The model under review builds one solid part; all positions refer to its coordinate system, in mm. Coordinates: 2 decimals unless noted, no trailing zeros. Write each loop counter-clockwise with the first axis right and the second up, starting at its lowest first coordinate (ties: lowest second). Pieces come first, ordered by that corner, then holes. Notation, with made-up numbers: M 70,19.25 L 117,19.25 A28 ccw 117,39.25 Z; hole C 50,66 d8. An arc over 180 degrees is marked long. Answer as a JSON object with one key per item and string values.
```python
from build123d import *

# Parameters (mm, degrees)
SKETCH1_W           = 150
SKETCH1_H           = 100
SKETCH1_R           = 2.5
SKETCH1_R_2         = 11.5
SKETCH1_R_3         = 1.5
SKETCH1_W_2         = 60
SKETCH1_H_2         = 45
BOSS_EXTRUDE1_DEPTH = 8
FILLET2_R           = 5
FILLET4_R           = 3


with BuildPart() as part:
    # Sketch1 → Boss-Extrude1 (new body)
    with BuildSketch(Plane(origin=(0, 0, 0), x_dir=(1, 0, 0), z_dir=(0, 1, 0))):
        Rectangle(SKETCH1_W, SKETCH1_H)
        with Locations(Location((-65, 40, 0), (0, 0, 270))):
            Circle(SKETCH1_R, mode=Mode.SUBTRACT)
        with Locations(Location((0, 40, 0), (0, 0, 270))):
            Circle(SKETCH1_R, mode=Mode.SUBTRACT)
        with Locations(Location((65, 40, 0), (0, 0, 270))):
            Circle(SKETCH1_R, mode=Mode.SUBTRACT)
        with Locations(Location((0, -40, 0), (0, 0, 270))):
            Circle(SKETCH1_R, mode=Mode.SUBTRACT)
        with Locations(Location((65, -40, 0), (0, 0, 270))):
            Circle(SKETCH1_R, mode=Mode.SUBTRACT)
        with Locations(Location((-65, -40, 0), (0, 0, 270))):
            Circle(SKETCH1_R, mode=Mode.SUBTRACT)
        with Locations(Location((-32.5, 0, 0), (0, 0, 270))):
            Circle(SKETCH1_R_2, mode=Mode.SUBTRACT)
        with Locations(Location((-50, 17.5, 0), (0, 0, 270))):
            Circle(SKETCH1_R_3, mode=Mode.SUBTRACT)
        with Locations(Location((-15, 17.5, 0), (0, 0, 270))):
            Circle(SKETCH1_R_3, mode=Mode.SUBTRACT)
        with Locations(Location((-15, -17.5, 0), (0, 0, 270))):
            Circle(SKETCH1_R_3, mode=Mode.SUBTRACT)
        with Locations(Location((-50, -17.5, 0), (0, 0, 270))):
            Circle(SKETCH1_R_3, mode=Mode.SUBTRACT)
        with Locations((27.5, 0)):
            Rectangle(SKETCH1_W_2, SKETCH1_H_2, mode=Mode.SUBTRACT)
    extrude(amount=BOSS_EXTRUDE1_DEPTH)

    # Fillet2
    fillet2_edges = [part.edges().sort_by_distance(p)[0] for p in [
        (-75, 4, 50),
        (-75, 4, -50),
        (75, 4, -50),
        (75, 4, 50),
    ]]
    fillet(fillet2_edges, radius=FILLET2_R)

    # Fillet4
    fillet4_edges = [part.edges().sort_by_distance(p)[0] for p in [
        (57.5, 4, 22.5),
        (57.5, 4, -22.5),
        (-2.5, 4, -22.5),
        (-2.5, 4, 22.5),
    ]]
    fillet(fillet4_edges, radius=FILLET4_R)


solid = part.part
```
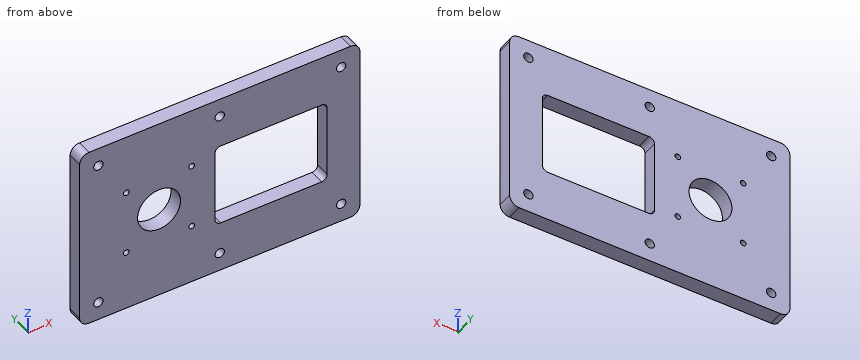
(1) Add section D-D on x = 65. Give the boundary of the cut face in (y, z), and give its area (3 significant figures).
Results list:
{"outline": "M 0,-50 L 8,-50 L 8,-42.5 L 0,-42.5 Z; M 0,-37.5 L 8,-37.5 L 8,37.5 L 0,37.5 Z; M 0,42.5 L 8,42.5 L 8,50 L 0,50 Z", "area": "720 mm²"}
(2) Wall thickness on line 1 along X through (y, z) = (2.5, 0); line 2 along X through (y, z) = (1.5, -40); line 3 along X through (y, z) = (7, 12.5): over which ranges is each line inside the solid? List them lowest first. Write a range as from..to.
Results list:
{"line 1": "-75..-44, -21..-2.5, 57.5..75", "line 2": "-75..-67.5, -62.5..-2.5, 2.5..62.5, 67.5..75", "line 3": "-75..-2.5, 57.5..75"}
(3) Add section A-A on z = 40. Give the boundary of the cut face in (x, y), and give its area (3 significant figures).
Results list:
{"outline": "M -75,0 L -67.5,0 L -67.5,8 L -75,8 Z; M -62.5,0 L -2.5,0 L -2.5,8 L -62.5,8 Z; M 2.5,0 L 62.5,0 L 62.5,8 L 2.5,8 Z; M 67.5,0 L 75,0 L 75,8 L 67.5,8 Z", "area": "1,080 mm²"}
(4) For pin 1 Ø4 at (x, z) = (-65, -40) entering from -Y, flat-tipped, find the tip position at first contact; note if it passes through.
Results list:
{"pin 1": "through"}
(5) Add section C-C on y = 1.25. Count the separate pieces of the cut face and the enclosed holes in it, and give its area (3 significant figures).
Results list:
{"separate pieces": "1", "enclosed holes": "12", "area": "11,700 mm²"}
(6) Add section B-B on x = 31. Give the boundary of the cut face in (y, z).
Results list:
{"outline": "M 0,-50 L 8,-50 L 8,-22.5 L 0,-22.5 Z; M 0,22.5 L 8,22.5 L 8,50 L 0,50 Z"}
